Autodesk Inventor part; units mm, degrees
ref_plane "YZ Plane" through (0, 0, 0) normal (1, 0, 0) x (0, 1, 0)
ref_plane "XZ Plane" through (0, 0, 0) normal (0, 1, 0) x (-1, 0, 0)
ref_plane "XY Plane" through (0, 0, 0) normal (0, 0, 1) x (1, 0, 0)
sketch "Szkic1" plane through (0, 0, 0) normal (1, 0, 0) x (0, 1, 0)
  line L0 (0, 0) -> (10.93, 0)
  line L1 (10.93, 0) -> (10.93, -100)
  line L2 (10.93, -100) -> (0, -100)
  line L3 (0, -100) -> (0, 0)
  dimension "d0" = 10.93
  dimension "d1" = 100
extrude "Wyciągnięcie proste1" add sketch "Szkic1" along normal blind 3
sketch "Szkic2" plane through (0, 0, -100) normal (0, -1, 0) x (1, 0, 0)
  line L0 (-5, 84) -> (-8.1113, 87.1113)
  line L1 (-5, 84) -> (-4.2222, 84.7778)
  line L2 (-8.1113, 87.1113) -> (-7.3335, 87.8891)
  line L3 (-2, 60) -> (-3.1388, 64.2501)
  line L4 (-2, 60) -> (-0.9375, 60.2847)
  line L5 (-3.1388, 64.2501) -> (-2.0763, 64.5348)
  line L6 (-3.1388, 35.7499) -> (-2, 40)
  line L7 (-3.1388, 35.7499) -> (-2.0763, 35.4652)
  line L8 (-2, 40) -> (-0.9375, 39.7153)
  line L9 (-8.1113, 12.8887) -> (-5, 16)
  line L10 (-8.1113, 12.8887) -> (-7.3335, 12.1109)
  line L11 (-5, 16) -> (-4.2222, 15.2222)
  line L12 (-30.0489, 4.1) -> (-25.6489, 4.1)
  line L13 (-30.0489, 4.1) -> (-30.0489, 3)
  line L14 (-25.6489, 4.1) -> (-25.6489, 3)
  line L15 (-1.7913, 81.5519) -> (-5, 78.3431)
  line L16 (-5, 78.3431) -> (-13.7681, 87.1113)
  line L17 (-13.7681, 87.1113) -> (-10.5594, 90.32)
  line L18 (-10.5594, 90.32) -> (185.0217, 443.1577)
  arc A0 (351.0464, 277.133) -> (185.0217, 443.1577) centre (-11.203, 80.9083) ccw
  line L19 (351.0464, 277.133) -> (-1.7913, 81.5519)
  arc A1 (402.9118, 49.2349) -> (342.1425, 276.0288) centre (-8.9178, 60.424) ccw
  line L20 (402.9118, 49.2349) -> (-0.4452, 56.2755)
  line L21 (-0.4452, 56.2755) -> (-4.8284, 55.101)
  line L22 (-4.8284, 55.101) -> (-8.0378, 67.0785)
  line L23 (-8.0378, 67.0785) -> (-3.6546, 68.253)
  line L24 (-3.6546, 68.253) -> (342.1425, 276.0288)
  arc A2 (342.1425, -176.0288) -> (402.9118, 50.7651) centre (-8.9178, 39.576) ccw
  line L25 (342.1425, -176.0288) -> (-3.6546, 31.747)
  line L26 (-3.6546, 31.747) -> (-8.0378, 32.9215)
  line L27 (-8.0378, 32.9215) -> (-4.8284, 44.899)
  line L28 (-4.8284, 44.899) -> (-0.4452, 43.7245)
  line L29 (-0.4452, 43.7245) -> (402.9118, 50.7651)
  arc A3 (185.0217, -343.1577) -> (351.0464, -177.133) centre (-11.203, 19.0917) ccw
  line L30 (185.0217, -343.1577) -> (-10.5594, 9.68)
  line L31 (-10.5594, 9.68) -> (-13.7681, 12.8887)
  line L32 (-13.7681, 12.8887) -> (-5, 21.6569)
  line L33 (-5, 21.6569) -> (-1.7913, 18.4481)
  line L34 (-1.7913, 18.4481) -> (351.0464, -177.133)
  line L35 (-25.6489, 3) -> (-30.0489, 3)
  line L36 (-0.9375, 39.7153) -> (-2.0763, 35.4652)
  line L37 (-7.3335, 87.8891) -> (-4.2222, 84.7778)
  line L38 (-2.0763, 64.5348) -> (-0.9375, 60.2847)
  line L39 (-4.2222, 15.2222) -> (-7.3335, 12.1109)
  point P0 (0, 100)
  point P1 (259.8393, 226.5761)
  point P2 (359.0779, 50)
  point P3 (259.8393, -126.5761)
  point P4 (343.886, -173.1639)
  point P5 (402.9318, 50)
  point P6 (343.886, 273.1639)
extrude "Wyciągnięcie proste2" cut sketch "Szkic2" against normal blind 5 contours L0 L2 L37 L1 | L3 L5 L38 L4 | L6 L8 L36 L7 | L9 L11 L39 L10 | L15 L16 L17 L18 A0 L19 A1 L24 | L24 A1 L19 | L19 A1 A2 L29 L20 L21 L22 L23 L24 | A2 L34 L25 L26 L27 L28 L29 L20 A1 | A1 L20 L29 A2 | L34 A3 L30 L31 L32 L33 L25 A2 | A2 L25 L34
sketch "Szkic3" plane through (3, 0, 0) normal (1, 0, 0) x (0, 0, -1)
  circle A0 centre (3.5, 7.9652) radius 2
  circle A1 centre (96.5, 7.9652) radius 2
  point P0 (0, 0)
hole "Otwór1" at (3, 7.9652, -3.5) at (3, 7.9652, -96.5) direction (-1, 0, 0) diameter 3.2 depth 5 tip angle 118 countersink diameter 5.5 countersink angle 90
properties part number "przod_kopia" material "Stal, odlew"
CAD build for the part. Positions are in the model's coordinates, mm. A direction names the side the tool comes from. Coordinates: 2 decimals unless noted, no trailing zeros. Order: outer loops, then holes, each group sorted by start corner. A loop starts at its lowest first (then second) coordinate and runs counter-clockwise, first axis right, second up.
(1) Pin check, flat tip, straight feed: pin 1 Ø1.5 at (x, z) = (1.5, -90) entering from -Y. Stop position of the tip, or through.
Solution:
pin 1: stops at y = 5
(2) Saw through at B-B, the plane z = -96.5. Write the cut outline in (x, y).
Solution:
outline: (0, 5) - (3, 5) - (3, 5.22) - (1.85, 6.37) - (0, 6.37) - close; (0, 9.57) - (1.85, 9.57) - (3, 10.72) - (3, 10.93) - (0, 10.93) - close
(3) Drill centre lines: L1, parallel to Z at x = 1.8, y = 8; L2, parallel to Y at x = 1.45, z = -96.5; L3, parallel to Z at x = 2.4, y = 1. Where is each one in solid material? Low to high.
Solution:
L1: z = -100 to -98.1, -94.9 to -5.1, -1.9 to 0
L2: y = 5 to 6.37, 9.57 to 10.93
L3: z = -83.88 to -71.89, -56.23 to -43.77, -28.11 to -16.12
(4) Mould opens along Z. For faces 1 (the face through (1, 5, -36)), 2 (the face through (1.521, 2.465, -16.612)), 3 (the face through (1, 0, -77)) say: released by +Z, released by -Z, zero draft, split by the parting line, or undercut.
Solution:
face 1: undercut
face 2: released by +Z
face 3: zero draft
(5) Saw through at A-A, the plane y = 2.5. Write the cut outline in (x, z), and give its area (3 significant figures).
Solution:
outline: (0, -82.54) - (3, -84.21) - (3, -72.25) - (0, -70.45) - close; (0, -56.27) - (3, -56.22) - (3, -43.78) - (0, -43.73) - close; (0, -29.55) - (3, -27.75) - (3, -15.79) - (0, -17.46) - close
area: 110 mm2
(6) Saw through at D-D, the plane z = -38. Write the cut outline in (x, y).
Solution:
outline: (0, 5) - (3, 5) - (3, 10.93) - (0, 10.93) - close
(7) Saw through at C-C, the plane x = 2.5. Write the cut outline in (y, z).
Solution:
outline: (0, -83.93) - (5, -83.93) - (5, -100) - (10.93, -100) - (10.93, 0) - (5, 0) - (5, -16.07) - (0, -16.07) - (0, -28.05) - (5, -28.05) - (5, -43.78) - (0, -43.78) - (0, -56.22) - (5, -56.22) - (5, -71.95) - (0, -71.95) - close; hole circle Ø4.5 at (7.97, -96.5); hole circle Ø4.5 at (7.97, -3.5)
(8) Which spindle directions (+Z, -Z, +X, -X, +Y, -Y) get a long thin tool onto all of the face, cutting with end or side? Do faces 4 (the face through (1.52, 2.46, -71.36)), 5 (the face through (1.479, 2.465, -83.365)), 6 (the face through (0, 7, -49)). Say none if no direction does.
Solution:
face 4: +X, -Y
face 5: -Z, -X, -Y
face 6: +Z, -Z, -X, +Y, -Y
